```python
from build123d import *

# Parameters (mm, degrees)
F1_DEPTH = 25.4
F3_DEPTH = 25.4


with BuildPart() as f1:
    # F0 (on Front) → F1 (new body, symmetric)
    with BuildSketch(Plane.XZ):
        with BuildLine():
            Line((-38.1, 232.930787788), (-9.525, 107.95))
            Line((-9.525, 107.95), (-9.525, 31.75))
            Line((-9.525, 31.75), (0, 0))
            Line((0, 0), (9.525, 31.75))
            Line((9.525, 31.75), (9.525, 107.95))
            Line((9.525, 107.95), (38.1, 232.930787788))
            add(Edge.make_bspline(
                [(38.1, 232.930787788), (38.1, 240.550787788), (37.5163115662, 241.1928509419), (37.3595791728, 248.750210884), (32.3169404592, 257.1928484496), (17.7830254248, 262.9110086651), (5.8041372503, 262.6187246427), (0, 262.8126600247)],
                knots=[0, 0, 0, 0, 0.1875465373, 0.3295066438, 0.5124130237, 0.74506917, 1, 1, 1, 1], degree=3))
            add(Edge.make_bspline(
                [(-38.1, 232.930787788), (-38.1, 240.550787788), (-37.5163115662, 241.1928509419), (-37.3595791728, 248.750210884), (-32.3169404592, 257.1928484496), (-17.7830254248, 262.9110086651), (-5.8041372503, 262.6187246427), (0, 262.8126600247)],
                knots=[0, 0, 0, 0, 0.1875465373, 0.3295066438, 0.5124130237, 0.74506917, 1, 1, 1, 1], degree=3))
        make_face()
    extrude(amount=F1_DEPTH, both=True)


with BuildPart() as f3:
    # F2 (on Right) → F3 (new body, symmetric)
    with BuildSketch(Plane.YZ):
        Polygon((29.1604775462, 70.3996203774), (0, 0), (-29.1604775462, 70.3996203774), (-87.4900998982, 70.3996203774), (-87.4900998982, -68.1293379466), (87.4900998982, -68.1293379466), (87.4900998982, 70.3996203774), align=None)
    extrude(amount=F3_DEPTH, both=True)


with BuildPart() as f1_1:
    add(f1.part)

    # F4: cut F3
    add(f3.part, mode=Mode.SUBTRACT)


solid = f1_1.part
```
Part model, mm, in its own coordinate system. A direction names the side the tool comes from. Coordinates: 2 decimals unless noted, no trailing zeros. Order: outer loops, then holes, each group sorted by start corner. A loop starts at its lowest first (then second) coordinate and runs counter-clockwise, first axis right, second up. Notation, with made-up numbers: (13.25, -13.5) -> (45.25, -13.5) arc R7 cw to (45.25, -3.5) -> close; hole circle Ø11 at (34.5, 73). An arc over 180 degrees is marked (long way). Put each result on its own line as item: value. Start each with the question number.
(1) Pin check, flat tips, straight feed: pin 1 Ø5 at (y, z) = (5.5, 154.5) entering from +X; pin 2 Ø12 at (x, y) = (28.5, 4.5) entering from +Z; pin 3 Ø8 at (y, z) = (-4.5, 219) entering from -X. Stop position of each tip, or through.
(2) Probe line 1 along X through (y, z) = (-16, 90.5) (3 decimals); line 2 along X through (y, z) = (10, 141.5); line 3 along Z through (x, y) = (-8.5, 23.5). List the from-to ranges inside material, lowest first. Write a range as [from, to].
(3) Band-saw the part on A-A (z = 64). Give the cut face in (x, y) (3 decimals).
(4) Band-saw the part on B-B (z = 26.5). Give the cut face in (x, y), then the cut area to 3 significant figures.
(5) Which spindle directions (+Z, -Z, +X, -X, +Y, -Y) get a long thin tool onto all of the face, cutting with end or side? Do faces 1 (the face through (9.525, 0, 69)), 2 (the face through (-9.525, 0, 70)), 3 (the face through (-1, 25.4, 186)). Say none if no direction does.
Determined:
1. pin 1: stops at x = 20.74
1. pin 2: stops at z = 260.61
1. pin 3: stops at x = -35.83
2. line 1: x = [-9.525, 9.525]
2. line 2: x = [-17.2, 17.2]
2. line 3: z = [56.73, 262.6]
3. outline: (-9.525, -25.4) -> (9.525, -25.4) -> (9.525, 25.4) -> (-9.525, 25.4) -> close
4. outline: (-7.95, -10.98) -> (7.95, -10.98) -> (7.95, 10.98) -> (-7.95, 10.98) -> close
4. area: 349 mm²
5. face 1: -Z, +X, +Y, -Y
5. face 2: -Z, -X, +Y, -Y
5. face 3: +Z, -Z, +X, -X, +Y
